Geometry: final body of the model. Coordinates: model frame, mm. Round coordinates to 2 decimals unless told otherwise and drop trailing zeros. Write each loop counter-clockwise with the first axis right and the second up, starting at its lowest first coordinate (ties: lowest second). Pieces come first, ordered by that corner, then holes. Notation, with made-up numbers: M -7.5,46.25 L 46.5,46.25 A28 ccw 46.5,73.25 Z; hole C -20,2.25 d3. An arc over 180 degrees is marked long. Use one line per item in the form item = value. Start each with the question number.
Item 1: Ray query, probe 1 along Y at (x, z) = (-5, 2.35); probe 2 along Y at (x, z) = (5, 1.9); probe 3 along X at (y, z) = (-16, 1.25). Return the intervals inside material, ascending.
Item 2: Section query B-B (z = 2.6). Return loops of the section in (x, y).
Item 3: Section query A-A (x = 5). Return loops of the section in (y, z).
Item 4: Pin query (flat end, axial travel): pin 1 Ø3.5 at (x, y) = (-5, 10) entering from +Z; pin 2 Ø1.8 at (x, y) = (-5, 16) entering from +Z. Return the tip coordinate at first contact, or that it passes through.
Item 5: Section query D-D (x = -5). Return loops of the section in (y, z), and give its area (3 significant figures).
Item 6: Section query C-C (y = -16). Return loops of the section in (x, z), and give its area (3 significant figures).
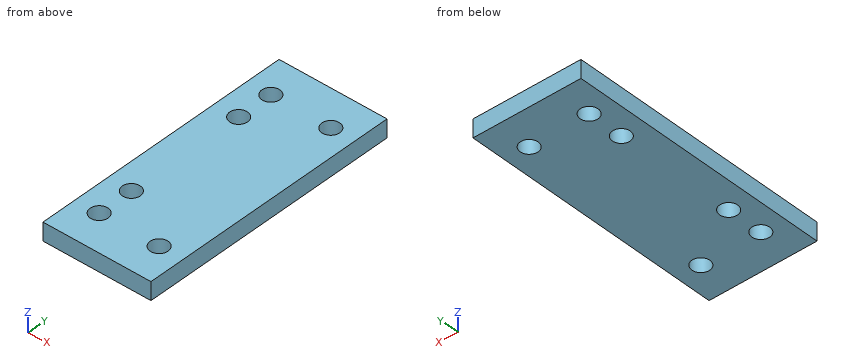
from build123d import *

# Parameters (mm, degrees)
F0_W     = 18
F0_H     = 44
F1_DEPTH = 3
F2_D     = 3


with BuildPart() as f1:
    # F0 (on Top) → F1 (new body)
    with BuildSketch(Plane.XY):
        Rectangle(F0_W, F0_H)
        Polygon((5, 16), (5, -16), (-5, -16), (-5, -10), (-5, 10), (-5, 16), align=None, mode=Mode.SUBTRACT)
        Polygon((-5, -16), (5, -16), (5, 16), (-5, 16), (-5, 10), (-5, -10), align=None)
    extrude(amount=F1_DEPTH)

    # F2 (through all)
    with Locations(Plane(origin=(0, 0, 0), x_dir=(1, 0, 0), z_dir=(0, 0, -1))):
        with Locations((-5, -16), (-5, 16), (-5, 10), (-5, -10), (5, -16), (5, 16)):
            Hole(F2_D / 2)


solid = f1.part
Working result:
q1.probe_1 = -22 to -17.5, -14.5 to -11.5, -8.5 to 8.5, 11.5 to 14.5, 17.5 to 22
q1.probe_2 = -22 to -17.5, -14.5 to 14.5, 17.5 to 22
q1.probe_3 = -9 to -6.5, -3.5 to 3.5, 6.5 to 9
q2.outline = M -9,-22 L 9,-22 L 9,22 L -9,22 Z; hole C -5,-16 d3; hole C -5,-10 d3; hole C -5,10 d3; hole C -5,16 d3; hole C 5,-16 d3; hole C 5,16 d3
q3.outline = M -22,0 L -17.5,0 L -17.5,3 L -22,3 Z; M -14.5,0 L 14.5,0 L 14.5,3 L -14.5,3 Z; M 17.5,0 L 22,0 L 22,3 L 17.5,3 Z
q4.pin_1 = 3
q4.pin_2 = through
q5.outline = M -22,0 L -17.5,0 L -17.5,3 L -22,3 Z; M -14.5,0 L -11.5,0 L -11.5,3 L -14.5,3 Z; M -8.5,0 L 8.5,0 L 8.5,3 L -8.5,3 Z; M 11.5,0 L 14.5,0 L 14.5,3 L 11.5,3 Z; M 17.5,0 L 22,0 L 22,3 L 17.5,3 Z
q5.area = 96.0 mm²
q6.outline = M -9,0 L -6.5,0 L -6.5,3 L -9,3 Z; M -3.5,0 L 3.5,0 L 3.5,3 L -3.5,3 Z; M 6.5,0 L 9,0 L 9,3 L 6.5,3 Z
q6.area = 36.0 mm²
